from build123d import *

# Parameters (mm, degrees)
F0_W     = 70
F0_H     = 70
F0_W_2   = 35
F0_H_2   = 35
F0_W_3   = 28
F0_H_3   = 28
F1_DEPTH = 3
F2_DEPTH = 130
F3_R     = 2
F5_DEPTH = 35
F6_R     = 3


with BuildPart() as f1:
    # F0 (on Top) → F1 (new body)
    with BuildSketch(Plane.XY):
        with Locations((-0.5, -3.077668637)):
            Rectangle(F0_W, F0_H)
        with Locations((0, -3.577668637)):
            Rectangle(F0_W_2, F0_H_2, mode=Mode.SUBTRACT)
        with Locations((0, -3.577668637)):
            Rectangle(F0_W_2, F0_H_2)
        with Locations((-0.5, -4.077668637)):
            Rectangle(F0_W_3, F0_H_3, mode=Mode.SUBTRACT)
        with Locations((-0.5, -4.077668637)):
            Rectangle(F0_W_3, F0_H_3)
    extrude(amount=-F1_DEPTH)

    # F0 (on Top) → F2 (join)
    with BuildSketch(Plane.XY):
        with Locations((0, -3.577668637)):
            Rectangle(F0_W_2, F0_H_2)
        with Locations((-0.5, -4.077668637)):
            Rectangle(F0_W_3, F0_H_3, mode=Mode.SUBTRACT)
    extrude(amount=-F2_DEPTH)

    # F3
    f3_edges = [f1.edges().sort_by_distance(p)[0] for p in [
        (-35.5, -38.077669, -1.5),
        (34.5, -38.077669, -1.5),
        (-35.5, 31.922331, -1.5),
        (34.5, 31.922331, -1.5),
    ]]
    fillet(f3_edges, radius=F3_R)

    # F4 (on face) → F5 (cut)
    with BuildSketch(Plane.XZ.offset(21.077668637)):
        with BuildLine():
            Line((3.4348594004, -130), (-0.5, -130))
            Line((-0.5, -130), (-0.5, -163))
            ThreePointArc((-0.5, -163), (2.0616616825, -163.9278851869), (3.4348594004, -166.2810552877))
            Line((3.4348594004, -166.2810552877), (3.4348594004, -130))
        make_face()
        with BuildLine():
            ThreePointArc((-0.5, -163), (-3.3284271247, -164.1715728753), (-4.5, -167))
            ThreePointArc((-4.5, -167), (-0.8609448701, -170.9836815637), (3.4348594004, -167.7189447123))
            Line((3.4348594004, -167.7189447123), (3.4348594004, -166.2810552877))
            ThreePointArc((3.4348594004, -166.2810552877), (2.0616616825, -163.9278851869), (-0.5, -163))
        make_face()
        with BuildLine():
            Line((-0.5, -130), (-4.5, -130))
            Line((-4.5, -130), (-4.5, -167))
            ThreePointArc((-4.5, -167), (-3.3284271247, -164.1715728753), (-0.5, -163))
            Line((-0.5, -163), (-0.5, -130))
        make_face()
        with BuildLine():
            Line((-4.5, -93), (-4.5, -130))
            Line((-4.5, -130), (-0.5, -130))
            Line((-0.5, -130), (-0.5, -97))
            ThreePointArc((-0.5, -97), (-3.3284271247, -95.8284271247), (-4.5, -93))
        make_face()
        with BuildLine():
            Line((-0.5, -97), (-0.5, -130))
            Line((-0.5, -130), (3.4348594004, -130))
            Line((3.4348594004, -130), (3.4348594004, -93.7189447123))
            ThreePointArc((3.4348594004, -93.7189447123), (2.0616616825, -96.0721148131), (-0.5, -97))
        make_face()
        with BuildLine():
            ThreePointArc((3.4348594004, -92.2810552877), (-0.8609448701, -89.0163184363), (-4.5, -93))
            ThreePointArc((-4.5, -93), (-3.3284271247, -95.8284271247), (-0.5, -97))
            ThreePointArc((-0.5, -97), (2.0616616825, -96.0721148131), (3.4348594004, -93.7189447123))
            Line((3.4348594004, -93.7189447123), (3.4348594004, -92.2810552877))
        make_face()
    extrude(amount=-F5_DEPTH, mode=Mode.SUBTRACT)

    # F6
    f6_edges = [f1.edges().sort_by_distance(p)[0] for p in [
        (17.5, -21.077669, -66.5),
        (17.5, 13.922331, -66.5),
        (-17.5, -21.077669, -66.5),
        (-17.5, 13.922331, -66.5),
    ]]
    fillet(f6_edges, radius=F6_R)


solid = f1.part
The listing builds one solid part. Answer for the finished solid, in the listing's coordinates (mm). A direction names the side the tool comes from. Round coordinates to 2 decimals unless told otherwise and drop trailing zeros. Order: outer loops, then holes, each group sorted by start corner. A loop starts at its lowest first (then second) coordinate and runs counter-clockwise, first axis right, second up. Notation, with made-up numbers: (53.25, 33) - (64.25, 33) arc R23 ccw to (64.25, 50) - close; hole circle Ø7 at (42.25, 83). An arc over 180 degrees is marked (long way). Write item = value, one per line. Start each with the question number.
1) Section C-C, the plane y = 0 is taken. Write down the section's boundary in (x, z).
2) For faces 4 (the flat face through (-1, -18.078, -66)), 5 (the cylindrical face through (-16.6, -20.22, -67.39)), 6 (the flat face through (-17.5, -4, -66)), 7 (the flat face through (-4.5, 12, -111)), determine the directions among +Z, -Z, +X, -X, +Y, -Y from which every point of the face is accessible in a straight line to the end or side of a thin tool.
3) Given pin 1 (14 mm diameter, centred on y = -3, z = -89.5, fed in from -X); pin 2 (22.5 mm diameter, centred on x = 4, z = -85.5, fed in from +Y); pin 3 (6 mm diameter, centred on x = 0, y = -26.5, fed in from -Z), each flat-ended and moving along its own axis, determine where each tip first touches the part or whether it passes through.
4) Section B-B, the plane z = -112.5 is taken. Write down the section's boundary in (x, y), plus the area to 3 significant figures.
5) Section A-A, the plane x = -7.5 is taken. Write down the section's boundary in (y, z), plus the area to 3 significant figures.
6) Straight lines are drawn through the part: L1, parallel to Y at x = 8.5, z = -8; L2, parallel to X at y = -16.5, z = -60.5; L3, parallel to Z at x = -18, y = 3.5. For each, find the intervals that lie inside material, in ascending order.
7) Section D-D, the plane z = -54.5 is taken. Write down the section's boundary in (x, y).
8) For a pull along Y with two mould halves and no side action, classify faces 1 (the flat face through (-4.5, -20, -111)), 2 (the flat face through (-1, -4, -3)), 3 (the flat face through (0, 13.922, -66)) as released by +Y, released by -Y, zero draft, split by the parting line, or undercut.
Results list:
q1.outline = (-35.5, -3) - (-17.5, -3) - (-17.5, -130) - (-14.5, -130) - (-14.5, -3) - (13.5, -3) - (13.5, -130) - (17.5, -130) - (17.5, -3) - (34.5, -3) - (34.5, 0) - (-35.5, 0) - close
q2.face_4 = -Z
q2.face_5 = -Z, -X, -Y
q2.face_6 = -Z, -X, +Y, -Y
q2.face_7 = -Z, +Y, -Y
q3.pin_1 = -17.5
q3.pin_2 = 13.92
q3.pin_3 = -3
q4.outline = (-17.5, -18.08) arc R3 ccw to (-14.5, -21.08) - (-4.5, -21.08) - (-4.5, -18.08) - (-14.5, -18.08) - (-14.5, 9.92) - (-4.5, 9.92) - (-4.5, 13.92) - (-14.5, 13.92) arc R3 ccw to (-17.5, 10.92) - close; (3.43, -21.08) - (14.5, -21.08) arc R3 ccw to (17.5, -18.08) - (17.5, 10.92) arc R3 ccw to (14.5, 13.92) - (3.43, 13.92) - (3.43, 9.92) - (13.5, 9.92) - (13.5, -18.08) - (3.43, -18.08) - close
q4.area = 378 mm^2
q5.outline = (-38.08, -3) - (-21.08, -3) - (-21.08, -130) - (-18.08, -130) - (-18.08, -3) - (9.92, -3) - (9.92, -130) - (13.92, -130) - (13.92, -3) - (31.92, -3) - (31.92, 0) - (-38.08, 0) - close
q5.area = 1,100 mm^2
q6.L1 = -21.08 to -18.08, 9.92 to 13.92
q6.L2 = -17.5 to -14.5, 13.5 to 17.5
q6.L3 = -3 to 0
q7.outline = (-17.5, -18.08) arc R3 ccw to (-14.5, -21.08) - (14.5, -21.08) arc R3 ccw to (17.5, -18.08) - (17.5, 10.92) arc R3 ccw to (14.5, 13.92) - (-14.5, 13.92) arc R3 ccw to (-17.5, 10.92) - close; hole (-14.5, -18.08) - (13.5, -18.08) - (13.5, 9.92) - (-14.5, 9.92) - close
q8.face_1 = zero draft
q8.face_2 = undercut
q8.face_3 = released by +Y
